from build123d import *

# Parameters (mm, degrees)
BOSS_EXTRUDE1_DEPTH = 12.7
FILLET1_R           = 6.604
FILLET2_R           = 6.604
SKETCH2_R           = 12.7
CUT_EXTRUDE1_DEPTH  = 1020.273904858
CUT_EXTRUDE3_DEPTH  = 1020.273904858
CUT_EXTRUDE4_DEPTH  = 1020.273904858
SKETCH6_R           = 3.3782
CUT_EXTRUDE5_DEPTH  = 1020.273904858
CUT_EXTRUDE6_DEPTH  = 1020.273904858
CUT_EXTRUDE7_DEPTH  = 1019.820731075
FILLET3_R           = 3.175


with BuildPart() as part:
    # Sketch1 → Boss-Extrude1 (new body)
    with BuildSketch(Plane(origin=(0, 0, 0), x_dir=(1, 0, 0), z_dir=(0, 1, 0))):
        Polygon((0, 0), (96.04375, 0), (96.04375, -190.5), (559.59375, -190.5), (559.59375, 0), (606.425, 0), (606.425, 819.15), (0, 819.15), align=None)
        with BuildLine():
            Line((19.05, 41.4782), (31.75, 41.4782))
            ThreePointArc((31.75, 41.4782), (35.1282, 38.1), (31.75, 34.7218))
            Line((31.75, 34.7218), (19.05, 34.7218))
            ThreePointArc((19.05, 34.7218), (15.6718, 38.1), (19.05, 41.4782))
        make_face(mode=Mode.SUBTRACT)
        with BuildLine():
            Line((19.05, 441.5282), (31.75, 441.5282))
            ThreePointArc((31.75, 441.5282), (35.1282, 438.15), (31.75, 434.7718))
            Line((31.75, 434.7718), (19.05, 434.7718))
            ThreePointArc((19.05, 434.7718), (15.6718, 438.15), (19.05, 441.5282))
        make_face(mode=Mode.SUBTRACT)
        with BuildLine():
            Line((31.75, 784.0218), (19.05, 784.0218))
            ThreePointArc((19.05, 784.0218), (15.6718, 787.4), (19.05, 790.7782))
            Line((19.05, 790.7782), (31.75, 790.7782))
            ThreePointArc((31.75, 790.7782), (35.1282, 787.4), (31.75, 784.0218))
        make_face(mode=Mode.SUBTRACT)
        with BuildLine():
            Line((577.85, 784.0218), (590.55, 784.0218))
            ThreePointArc((590.55, 784.0218), (593.9282, 787.4), (590.55, 790.7782))
            Line((590.55, 790.7782), (577.85, 790.7782))
            ThreePointArc((577.85, 790.7782), (574.4718, 787.4), (577.85, 784.0218))
        make_face(mode=Mode.SUBTRACT)
        with BuildLine():
            Line((590.55, 441.5282), (577.85, 441.5282))
            ThreePointArc((577.85, 441.5282), (574.4718, 438.15), (577.85, 434.7718))
            Line((577.85, 434.7718), (590.55, 434.7718))
            ThreePointArc((590.55, 434.7718), (593.9282, 438.15), (590.55, 441.5282))
        make_face(mode=Mode.SUBTRACT)
        with BuildLine():
            Line((590.55, 41.4782), (577.85, 41.4782))
            ThreePointArc((577.85, 41.4782), (574.4718, 38.1), (577.85, 34.7218))
            Line((577.85, 34.7218), (590.55, 34.7218))
            ThreePointArc((590.55, 34.7218), (593.9282, 38.1), (590.55, 41.4782))
        make_face(mode=Mode.SUBTRACT)
    extrude(amount=BOSS_EXTRUDE1_DEPTH)

    # Fillet1
    fillet1_edges = [part.edges().sort_by_distance(p)[0] for p in [
        (559.59375, 6.35, 0),
        (96.04375, 6.35, 0),
    ]]
    fillet(fillet1_edges, radius=FILLET1_R)

    # Fillet2
    fillet2_edges = [part.edges().sort_by_distance(p)[0] for p in [
        (0, 6.35, -819.15),
        (606.425, 6.35, -819.15),
        (606.425, 6.35, 0),
        (559.59375, 6.35, 190.5),
        (96.04375, 6.35, 190.5),
        (0, 6.35, 0),
    ]]
    fillet(fillet2_edges, radius=FILLET2_R)

    # Sketch2 → Cut-Extrude1 (cut, through all)
    with BuildSketch(Plane(origin=(0, 12.7, 0), x_dir=(1, 0, 0), z_dir=(0, 1, 0))):
        with Locations(Location((47.625, 483.87, 0), (0, 0, 270))):
            Circle(SKETCH2_R)
        with BuildLine():
            Line((606.425, 505.867045256), (606.425, 461.872954744))
            ThreePointArc((606.425, 461.872954744), (604.723522628, 468.222954744), (600.075, 472.871477372))
            ThreePointArc((600.075, 472.871477372), (593.725, 483.87), (600.075, 494.868522628))
            ThreePointArc((600.075, 494.868522628), (604.723522628, 499.517045256), (606.425, 505.867045256))
        make_face()
    extrude(amount=-CUT_EXTRUDE1_DEPTH, mode=Mode.SUBTRACT)

    # Sketch4 → Cut-Extrude3 (cut, through all)
    with BuildSketch(Plane.XZ):
        with BuildLine():
            Line((350.8375, -527.05), (350.8375, -549.275))
            ThreePointArc((350.8375, -549.275), (327.025, -573.0875), (303.2125, -549.275))
            Line((303.2125, -549.275), (303.2125, -527.05))
            ThreePointArc((303.2125, -527.05), (327.025, -503.2375), (350.8375, -527.05))
        make_face()
        with BuildLine():
            Line((350.8375, 0), (350.8375, -22.225))
            ThreePointArc((350.8375, -22.225), (327.025, -46.0375), (303.2125, -22.225))
            Line((303.2125, -22.225), (303.2125, 0))
            ThreePointArc((303.2125, 0), (327.025, 23.8125), (350.8375, 0))
        make_face()
    extrude(amount=-CUT_EXTRUDE3_DEPTH, mode=Mode.SUBTRACT)

    # Sketch5 → Cut-Extrude4 (cut, through all)
    with BuildSketch(Plane.XZ):
        with BuildLine():
            Line((320.675, -466.725), (320.675, -82.55))
            ThreePointArc((320.675, -82.55), (327.025, -76.2), (333.375, -82.55))
            Line((333.375, -82.55), (333.375, -466.725))
            ThreePointArc((333.375, -466.725), (327.025, -473.075), (320.675, -466.725))
        make_face()
    extrude(amount=-CUT_EXTRUDE4_DEPTH, mode=Mode.SUBTRACT)

    # Sketch6 → Cut-Extrude5 (cut, through all)
    with BuildSketch(Plane.XZ):
        with Locations(Location((354.0125, -274.6375, 0), (0, 0, 270))):
            Circle(SKETCH6_R)
        with Locations(Location((354.0125, -427.0375, 0), (0, 0, 270))):
            Circle(SKETCH6_R)
        with Locations(Location((354.0125, -122.2375, 0), (0, 0, 90))):
            Circle(SKETCH6_R)
        with Locations(Location((300.0375, -427.0375, 0), (0, 0, 90))):
            Circle(SKETCH6_R)
        with Locations(Location((300.0375, -274.6375, 0), (0, 0, 90))):
            Circle(SKETCH6_R)
        with Locations(Location((300.0375, -122.2375, 0), (0, 0, 270))):
            Circle(SKETCH6_R)
    extrude(amount=-CUT_EXTRUDE5_DEPTH, mode=Mode.SUBTRACT)

    # Sketch7 → Cut-Extrude6 (cut, through all)
    with BuildSketch(Plane.XZ):
        with BuildLine():
            ThreePointArc((605.663, -812.546), (603.728733183, -817.215733183), (599.059, -819.15))
            Line((599.059, -819.15), (599.821, -819.15))
            ThreePointArc((599.821, -819.15), (604.490733183, -817.215733183), (606.425, -812.546))
            Line((606.425, -812.546), (606.425, -505.867045256))
            ThreePointArc((606.425, -505.867045256), (604.723522628, -499.517045256), (600.075, -494.868522628))
            ThreePointArc((600.075, -494.868522628), (604.165699913, -498.959222541), (605.663, -504.547222541))
            Line((605.663, -504.547222541), (605.663, -812.546))
        make_face()
        with BuildLine():
            ThreePointArc((0.762, -812.546), (2.696266817, -817.215733183), (7.366, -819.15))
            Line((7.366, -819.15), (6.604, -819.15))
            ThreePointArc((6.604, -819.15), (1.934266817, -817.215733183), (0, -812.546))
            Line((0, -812.546), (0, -6.604))
            ThreePointArc((0, -6.604), (1.934266817, -1.934266817), (6.604, 0))
            Line((6.604, 0), (7.366, 0))
            ThreePointArc((7.366, 0), (2.696266817, -1.934266817), (0.762, -6.604))
            Line((0.762, -6.604), (0.762, -812.546))
        make_face()
        with BuildLine():
            ThreePointArc((605.663, -462.330859906), (604.07096336, -468.487413325), (599.694, -473.100429953))
            ThreePointArc((599.694, -473.100429953), (599.883498256, -472.98428666), (600.075, -472.871477372))
            ThreePointArc((600.075, -472.871477372), (604.723522628, -468.222954744), (606.425, -461.872954744))
            Line((606.425, -461.872954744), (606.425, -6.604))
            ThreePointArc((606.425, -6.604), (604.490733183, -1.934266817), (599.821, 0))
            Line((599.821, 0), (599.059, 0))
            ThreePointArc((599.059, 0), (603.728733183, -1.934266817), (605.663, -6.604))
            Line((605.663, -6.604), (605.663, -462.330859906))
        make_face()
    extrude(amount=-CUT_EXTRUDE6_DEPTH, mode=Mode.SUBTRACT)

    # Sketch8 → Cut-Extrude7 (cut, through all)
    with BuildSketch(Plane.XZ):
        with BuildLine():
            ThreePointArc((595.884, -819.15), (600.553733183, -817.215733183), (602.488, -812.546))
            Line((602.488, -812.546), (602.488, -6.604))
            ThreePointArc((602.488, -6.604), (600.553733183, -1.934266817), (595.884, 0))
            Line((595.884, 0), (599.059, 0))
            ThreePointArc((599.059, 0), (603.728733183, -1.934266817), (605.663, -6.604))
            Line((605.663, -6.604), (605.663, -812.546))
            ThreePointArc((605.663, -812.546), (603.728733183, -817.215733183), (599.059, -819.15))
            Line((599.059, -819.15), (595.884, -819.15))
        make_face()
        with BuildLine():
            Line((0.762, -6.604), (0.762, -812.546))
            ThreePointArc((0.762, -812.546), (2.696266817, -817.215733183), (7.366, -819.15))
            Line((7.366, -819.15), (16.891, -819.15))
            ThreePointArc((16.891, -819.15), (12.221266817, -817.215733183), (10.287, -812.546))
            Line((10.287, -812.546), (10.287, -6.604))
            ThreePointArc((10.287, -6.604), (12.221266817, -1.934266817), (16.891, 0))
            Line((16.891, 0), (7.366, 0))
            ThreePointArc((7.366, 0), (2.696266817, -1.934266817), (0.762, -6.604))
        make_face()
    extrude(amount=-CUT_EXTRUDE7_DEPTH, mode=Mode.SUBTRACT)

    # Fillet3
    fillet3_edges = [part.edges().sort_by_distance(p)[0] for p in [
        (602.488, 6.35, -470.731120318),
        (602.488, 6.35, -496.744211904),
    ]]
    fillet(fillet3_edges, radius=FILLET3_R)


solid = part.part
Work out the finished part from the listing and answer in its coordinate system (mm). A direction names the side the tool comes from. Round coordinates to 2 decimals unless told otherwise and drop trailing zeros. Loops run counter-clockwise (first coordinate to the right, second up) from the corner with the lowest first, then second, coordinate; pieces in that order, holes last. Notation, with made-up numbers: M 85,5.25 L 110,5.25 A19 cw 110,37.25 Z; hole C 45,29.25 d4. An arc over 180 degrees is marked long. One line per question, with ' | ' between items. Start each with the question number.
(1) For a pull along X with two mould halves and no side action, classify faces 3 (the face through (302, 0, -321)), 4 (the face through (326.501, 6.261, -503.243)) as released by +X, released by -X, zero draft, split by the parting line, or undercut.
(2) A cutting plane is placed at A-A on z = -483.87. Write down the section's boundary in (x, y) (3 decimals), plus the area to 3 significant figures.
(3) Find the intervals of material crossed by line 1 (X direction, y = 6.5, z = -346) (3 decimals); line 2 (X direction, y = 3.75, z = -20); line 3 (X direction, y = 1.5, z = -124.5) (3 decimals), in increasing order.
(4) A cutting plane is placed at B-B on z = 104.5. Write down the section's boundary in (x, y), plus the area to 3 significant figures.
(5) A cutting plane is placed at C-C on y = 10.75. Give the number of separate pieces and of enclosed holes in the cut face, plus the area to 3 significant figures.
(6) Flat-ended cylindrical pins translate along their axes: pin 1 Ø5.5 at (x, z) = (300.04, -427.04) entering from +Y; pin 2 Ø6.5 at (x, y) = (582, 6) entering from +Z. Find the tip coordinate at first contact, or state that the pin passes through.
(7) A tool of negligible diameter and unlimited length cuts with its end or side. For faces 1 (the face through (302, 12.7, -321)), 2 (the face through (327.55, 6.26, -573.08)), from which of +Z, -Z, +X, -X, +Y, -Y can it reach the whole face along a straight path? Write none if from no direction.
Geometry check:
1) face 3: zero draft | face 4: undercut
2) outline: M 10.287,0 L 34.925,0 L 34.925,12.7 L 10.287,12.7 Z; M 60.325,0 L 593.725,0 L 593.725,12.7 L 60.325,12.7 Z | area: 7,090 mm²
3) line 1: x = 10.287 to 320.675, 333.375 to 602.488 | line 2: x = 10.29 to 303.21, 350.84 to 602.49 | line 3: x = 10.287 to 297.529, 302.546 to 320.675, 333.375 to 351.504, 356.521 to 602.488
4) outline: M 96.04,0 L 559.59,0 L 559.59,12.7 L 96.04,12.7 Z | area: 5,890 mm²
5) separate pieces: 1 | enclosed holes: 16 | area: 561,000 mm²
6) pin 1: passes through | pin 2: stops at z = 0
7) face 1: +Z, -Z, +X, -X, +Y | face 2: +Y, -Y
